Autodesk Inventor part; units mm, degrees
ref_plane "YZ Plane" through (0, 0, 0) normal (1, 0, 0) x (0, 1, 0)
ref_plane "XZ Plane" through (0, 0, 0) normal (0, 1, 0) x (-1, 0, 0)
ref_plane "XY Plane" through (0, 0, 0) normal (0, 0, 1) x (1, 0, 0)
sketch "스케치1" plane through (0, 0, 0) normal (0, 0, 1) x (1, 0, 0)
  line L0 (0, 0) -> (150, 0)
  line L1 (150, 0) -> (150, 141.5)
  line L2 (150, 141.5) -> (0, 141.5)
  line L3 (0, 141.5) -> (0, 0)
  dimension "d0" = 150
  dimension "d1" = 141.5
extrude "돌출1" add sketch "스케치1" along normal blind 86.5
sketch "스케치2" plane through (0, 0, 86.5) normal (0, 0, 1) x (1, 0, 0)
  line L0 (150, 0) -> (150, 141.5)
  line L1 (137, 18.25) -> (32, 18.25) construction
  line L2 (32, 18.25) -> (32, 123.25) construction
  line L3 (32, 123.25) -> (137, 123.25) construction
  line L4 (137, 123.25) -> (137, 18.25) construction
  line L5 (137, 18.25) -> (32, 123.25) construction
  line L6 (32, 18.25) -> (137, 123.25) construction
  circle A0 centre (32, 123.25) radius 2.5
  circle A1 centre (32, 18.25) radius 2.5
  circle A2 centre (137, 18.25) radius 2.5
  circle A3 centre (137, 123.25) radius 2.5
  point P0 (84.5, 70.75)
  point P1 (32, 70.75)
  point P2 (0, 70.75)
  dimension "d4" = 105
  dimension "d5" = 105
  dimension "d7" = 13
  dimension "d9" = 5
  dimension "d12" = 360
extrude "돌출2" cut sketch "스케치2" against normal blind 5
sketch "스케치3" plane through (0, 0, 86.5) normal (0, 0, 1) x (1, 0, 0)
  circle A0 centre (32, 123.25) radius 2.5 construction
  circle A1 centre (137, 18.25) radius 2.5 construction
  line L0 (32, 123.25) -> (137, 123.25) construction
  line L1 (137, 123.25) -> (137, 18.25) construction
  line L2 (137, 18.25) -> (32, 18.25) construction
  line L3 (32, 18.25) -> (32, 123.25) construction
  line L4 (84.5, 123.25) -> (84.5, 70.75) construction
  line L5 (84.5, 70.75) -> (137, 70.75) construction
  line L6 (119.3236, 11.75) -> (49.6764, 11.75)
  line L7 (25.5, 35.9264) -> (25.5, 105.5736)
  line L8 (49.6764, 129.75) -> (119.3236, 129.75)
  line L9 (143.5, 105.5736) -> (143.5, 35.9264)
  line L10 (143.5, 11.75) -> (25.5, 129.75) construction
  line L11 (25.5, 11.75) -> (143.5, 129.75) construction
  line L12 (119.3236, 129.75) -> (143.5, 105.5736)
  line L13 (25.5, 105.5736) -> (49.6764, 129.75)
  line L14 (49.6764, 11.75) -> (25.5, 35.9264)
  line L15 (143.5, 35.9264) -> (119.3236, 11.75)
  point P0 (150, 141.5)
  dimension "d28" = 360
  dimension "d16" = 90
  dimension "d21" = 118
  dimension "d22" = 45
  dimension "d24" = 45
  dimension "d25" = 30
extrude "돌출3" cut sketch "스케치3" against normal blind 10
sketch "스케치4" plane through (0, 141.5, 0) normal (0, 1, 0) x (1, 0, 0)
  line L0 (20.5008, -63.1326) -> (20.5008, -47.8147)
  line L1 (20.5008, -47.8147) -> (50.8737, -47.8147)
  line L2 (50.8737, -47.8147) -> (50.8737, -63.1326)
  line L3 (50.8737, -63.1326) -> (42.1805, -66.6205)
  line L4 (42.1805, -66.6205) -> (29.194, -66.6205)
  line L5 (29.194, -66.6205) -> (20.5008, -63.1326)
  point P0 (35.6872, -66.6205)
  point P1 (35.6872, -47.8147)
extrude "돌출4" cut sketch "스케치4" against normal blind 10
properties part number "파워서플라이"
CAD build for the part. Positions are in the model's coordinates, mm. A direction names the side the tool comes from. Coordinates: 2 decimals unless noted, no trailing zeros. Write each loop counter-clockwise with the first axis right and the second up, starting at its lowest first coordinate (ties: lowest second). Pieces come first, ordered by that corner, then holes.
(1) Cut at B-B, the plane x = 92. List the corners of the cut face in (y, z), and give its area (3 significant figures).
(2) Cut at A-A, the plane y = 61.5. List the corners of the cut face in (x, z), and give its area (3 significant figures).
(3) Cut at D-D, the plane y = 18.25. List the corners of the cut face in (x, z), and give its area (3 significant figures).
(4) Drill centre lines: probe 1 along Y at (x, z) = (137, 83); probe 2 along X at (y, z) = (18, 82); probe 3 along X at (y, z) = (123, 84). Where is each one in solid material? Low to high.
(5) Flat gauge pin, fed straight in: pin 1 (4.5 mm diameter, centred on x = 137, y = 18.25, fed in from +Z). Where does the tip first touch, or does it go through?
(6) Two-plate mould, pull along Y, no slides. Class faces 4 (the face through (143.5, 71, 82)), 5 (the face through (24.91, 136.57, 64.9)), 6 (the face through (84, 72, 76.5)), 7 (the face through (35, 131.5, 57)): +Y half, -Y half, draft (parallel to the pull), parting line (faces both ways), or undercut.
(7) Cut at C-C, the plane x = 32. List the corners of the cut face in (y, z).
(8) 3-axis set-ups, long thin cutter, end or side, ignore diameter. For faces 1 (the face through (36, 137, 66.62)), 2 (the face through (37.757, 23.669, 81.57)), 3 (the face through (0, 72, 43)): which of +Z, -Z, +X, -X, +Y, -Y reach the whole face in a straight line?
Geometry says:
1. outline: (0, 0) - (141.5, 0) - (141.5, 86.5) - (129.75, 86.5) - (129.75, 76.5) - (11.75, 76.5) - (11.75, 86.5) - (0, 86.5) - close
1. area: 11,100 mm2
2. outline: (0, 0) - (150, 0) - (150, 86.5) - (143.5, 86.5) - (143.5, 76.5) - (25.5, 76.5) - (25.5, 86.5) - (0, 86.5) - close
2. area: 11,800 mm2
3. outline: (0, 0) - (150, 0) - (150, 86.5) - (139.5, 86.5) - (139.5, 81.5) - (134.5, 81.5) - (134.5, 86.5) - (125.82, 86.5) - (125.82, 76.5) - (43.18, 76.5) - (43.18, 86.5) - (34.5, 86.5) - (34.5, 81.5) - (29.5, 81.5) - (29.5, 86.5) - (0, 86.5) - close
3. area: 12,100 mm2
4. probe 1: y = 0 to 15.75, 20.75 to 29.43, 112.07 to 120.75, 125.75 to 141.5
4. probe 2: x = 0 to 29.51, 34.49 to 43.43, 125.57 to 134.51, 139.49 to 150
4. probe 3: x = 0 to 29.51, 34.49 to 42.93, 126.07 to 134.51, 139.49 to 150
5. pin 1: stops at z = 81.5
6. face 4: undercut
6. face 5: draft
6. face 6: undercut
6. face 7: +Y half
7. outline: (0, 0) - (141.5, 0) - (141.5, 47.81) - (131.5, 47.81) - (131.5, 66.62) - (141.5, 66.62) - (141.5, 86.5) - (125.75, 86.5) - (125.75, 81.5) - (120.75, 81.5) - (120.75, 86.5) - (112.07, 86.5) - (112.07, 76.5) - (29.43, 76.5) - (29.43, 86.5) - (20.75, 86.5) - (20.75, 81.5) - (15.75, 81.5) - (15.75, 86.5) - (0, 86.5) - close
8. face 1: +Y
8. face 2: +Z
8. face 3: +Z, -Z, -X, +Y, -Y
